from build123d import *

# Parameters (mm, degrees)
SKETCH2_R           = 8
SKETCH2_R_2         = 7
BOSS_EXTRUDE2_DEPTH = 88.69527324
M2_TAPPED_HOLE1_D   = 1.6
M2_TAPPED_HOLE2_D   = 1.6


with BuildPart() as part:
    # Sketch2 → Boss-Extrude2 (new body)
    with BuildSketch(Plane(origin=(0, 0, 0), x_dir=(1, 0, 0), z_dir=(0, 1, 0))):
        Circle(SKETCH2_R)
        Circle(SKETCH2_R_2, mode=Mode.SUBTRACT)
    extrude(amount=BOSS_EXTRUDE2_DEPTH)

    # M2 Tapped Hole1 (through all)
    with Locations(Plane(origin=(8, 0, 0), x_dir=(0, 0, -1), z_dir=(1, 0, 0))):
        with Locations((0, 78.27915224)):
            Hole(M2_TAPPED_HOLE1_D / 2)

    # M2 Tapped Hole2 (through all)
    with Locations(Plane(origin=(8, 0, 0), x_dir=(0, 0, -1), z_dir=(1, 0, 0))):
        with Locations((0, 11)):
            Hole(M2_TAPPED_HOLE2_D / 2)


solid = part.part
Source: CAD feature listing. Evaluate the final solid. Frame: model axes, mm. Round coordinates to 2 decimals unless told otherwise and drop trailing zeros. Loops run counter-clockwise (first coordinate to the right, second up) from the corner with the lowest first, then second, coordinate; pieces in that order, holes last. Notation, with made-up numbers: (87.25, 35) - (120.25, 35) arc R21 ccw to (120.25, 43) - close; hole circle Ø4 at (-12.5, -33). An arc over 180 degrees is marked (long way). Write item = value, one per line. Start each with the question number.
(1) Section query D-D, the plane y = 38. Output: boundary loops of the cut face in (x, z).
(2) Pin query (flat end, axial travel): pin 1 (1.4 mm diameter, centred on y = 11, z = 0, fed in from +X); pin 2 (2 mm diameter, centred on x = 1, y = 50.5, fed in from -Z). Return the tip coordinate at first contact, or that it passes through.
(3) Pull-direction query (X, two-part tool) for faces 1 (the face through (6.466, 43.727, 2.681)), 2 (the face through (-1.73, 43.73, 7.81)), 3 (the face through (-7.484, 11.793, -0.104)); classes: +X half, -X half, draft (parallel to the pull), parting line (faces both ways), or undercut.
(4) Section query B-B, the plane z = 0. Output: boundary loops of the cut face in (x, y).
(5) Section query C-C, the plane y = 11. Output: boundary loops of the cut face in (x, z), plus the area to 3 significant figures.
(6) Section query A-A, the plane x = 0. Output: boundary loops of the cut face in (y, z).
(7) Ray query, line 1 along Y through (x, z) = (-7.5, 0); line 2 along Z through (x, y) = (-6.25, 64.5); line 3 along X through (y, z) = (57, 0). Return the intervals inside material, ascending. Write a range as from..to.
Conclusion:
q1.outline = circle Ø16 at (0, 0); hole circle Ø14 at (0, 0)
q2.pin_1 = through
q2.pin_2 = -8
q3.face_1 = undercut
q3.face_2 = parting line
q3.face_3 = draft
q4.outline = (-8, 0) - (-7, 0) - (-7, 10.2) - (-8, 10.2) - close; (-8, 11.8) - (-7, 11.8) - (-7, 77.48) - (-8, 77.48) - close; (-8, 79.08) - (-7, 79.08) - (-7, 88.7) - (-8, 88.7) - close; (7, 0) - (8, 0) - (8, 10.2) - (7, 10.2) - close; (7, 11.8) - (8, 11.8) - (8, 77.48) - (7, 77.48) - close; (7, 79.08) - (8, 79.08) - (8, 88.7) - (7, 88.7) - close
q5.outline = (-7.96, -0.8) arc R8 ccw to (7.96, -0.8) - (6.95, -0.8) arc R7 cw to (-6.95, -0.8) - close; (-7.96, 0.8) - (-6.95, 0.8) arc R7 cw to (6.95, 0.8) - (7.96, 0.8) arc R8 ccw to start
q5.area = 43.9 mm2
q6.outline = (0, -8) - (88.7, -8) - (88.7, -7) - (0, -7) - close; (0, 7) - (88.7, 7) - (88.7, 8) - (0, 8) - close
q7.line_1 = 0..10.2, 11.8..77.48, 79.08..88.7
q7.line_2 = -4.99..-3.15, 3.15..4.99
q7.line_3 = -8..-7, 7..8
